Verification items for the finished model (mm, model axes). A direction names the side the tool comes from. Round coordinates to 2 decimals unless told otherwise and drop trailing zeros. Order: outer loops, then holes, each group sorted by start corner. A loop starts at its lowest first (then second) coordinate and runs counter-clockwise, first axis right, second up.
Autodesk Fusion 360 part; units mm, degrees
sketch "Sketch1" plane through (0, 0, 0) normal (0, 0, 1) x (1, 0, 0)
  line L0 (0, 0) -> (16.5, 0)
  line L1 (16.5, 0) -> (16.5, 1.6)
  line L2 (16.5, 1.6) -> (0, 1.6)
  line L3 (0, 1.6) -> (0, 0)
  line L4 (2.75, 1.6) -> (13.75, 1.6)
  line L5 (13.75, 1.6) -> (13.75, 7.6)
  line L6 (13.75, 7.6) -> (2.75, 7.6)
  line L7 (2.75, 7.6) -> (2.75, 1.6)
  dimension "d1" = 16.5
  dimension "d2" = 1.6
  dimension "d3" = 11
  dimension "d4" = 6
  dimension "d5" = 2.75
extrude "Extrude1" add sketch "Sketch1" along normal blind 10
sketch "Sketch2" plane through (2.75, 0, 0) normal (-1, 0, 0) x (0, -1, 0)
  line L0 (-7.6, 0) -> (-1.6, 0)
  line L1 (-1.6, 0) -> (-1.6, 10)
  line L2 (-1.6, 10) -> (-7.6, 10)
  line L3 (-7.6, 10) -> (-7.6, 0)
  line L4 (-7.6, 10) -> (-11.6, 10)
  line L5 (-11.6, 10) -> (-7.6, 3.0718)
  line L6 (-11.6, 10) -> (-3.6, 10) construction
  dimension "d8" = 4
  dimension "d9" = 60
extrude "Extrude2" add sketch "Sketch2" against normal blind 11 contours L3 L4 L5
fillet "Fillet1" radius 0.25 8 edges at (2.75, 6.6, 10) (1.375, 1.6, 10) (0, 0.8, 10) (8.25, 0, 10) (16.5, 0.8, 10) (15.125, 1.6, 10) (13.75, 6.6, 10) (8.25, 11.6, 10)
equation "d5 = ( ( 16.5 - 11 ) / 2 ) * 1 mm"
1) Tool access check on faces 1 (the flat face through (8, 0, 5)), 2 (the flat face through (15, 1.6, 5)), 3 (the flat face through (2.75, 5, 6)), 4 (the flat face through (8, 7.6, 2)). Record the directions out of +Z, -Z, +X, -X, +Y, -Y that give a thin tool (end or side, any length) a straight path to the whole face; none if there is none.
2) Sectioned sample at D-D on y = 2. Record the cut outline in (x, z), then the cut area to 3 significant figures.
3) Go/stop test with flat-tipped pins: pin 1 Ø5 at (x, z) = (10, 7) entering from +Y; pin 2 Ø3 at (y, z) = (6, 2.5) entering from +X; pin 3 Ø0.8 at (x, z) = (0.5, 7.5) entering from +Y. Record where each tip stops, or that it passes through.
4) Sectioned sample at A-A on z = 9.25. Record the cut outline in (x, y), then the cut area to 3 significant figures.
5) Sectioned sample at C-C on z = 1.75. Record the cut outline in (x, y), then the cut area to 3 significant figures.
6) Scan lines: probe 1 along X at (y, z) = (1.75, 7.25); probe 2 along Y at (x, z) = (16, 0.75); probe 3 along Y at (x, z) = (6.5, 3). Record each from-to range of solid material in increasing order.
Returned:
1. face 1: +Z, -Z, +X, -X, -Y
1. face 2: +Z, -Z, +X, +Y
1. face 3: +Z, -Z, -X, +Y
1. face 4: -Z, +X, -X, +Y
2. outline: (2.75, 0) - (13.75, 0) - (13.75, 9.75) arc R0.25 ccw to (13.5, 10) - (3, 10) arc R0.25 ccw to (2.75, 9.75) - close
2. area: 110 mm2
3. pin 1: stops at y = 11.31
3. pin 2: stops at x = 13.75
3. pin 3: stops at y = 1.6
4. outline: (0, 0) - (16.5, 0) - (16.5, 1.6) - (13.75, 1.6) - (13.75, 11.17) - (2.75, 11.17) - (2.75, 1.6) - (0, 1.6) - close
4. area: 132 mm2
5. outline: (0, 0) - (16.5, 0) - (16.5, 1.6) - (13.75, 1.6) - (13.75, 7.6) - (2.75, 7.6) - (2.75, 1.6) - (0, 1.6) - close
5. area: 92.4 mm2
6. probe 1: x = 2.75 to 13.75
6. probe 2: y = 0 to 1.6
6. probe 3: y = 0 to 7.6
